Check sheet for the modelled part. Datum: model origin and axes. Units: mm. A direction names the side the tool comes from. Round coordinates to 2 decimals unless told otherwise and drop trailing zeros. Write each loop counter-clockwise with the first axis right and the second up, starting at its lowest first coordinate (ties: lowest second). Pieces come first, ordered by that corner, then holes. Notation, with made-up numbers: M 63.5,31.5 L 109.5,31.5 A21 ccw 109.5,52.5 Z; hole C 65.25,-23 d1. An arc over 180 degrees is marked long. One line per item, written item: value.
from build123d import *

# Parameters (mm, degrees)
F2_DEPTH = 3.175
F3_DEPTH = 3.175
F4_R     = 7.203715
F5_DEPTH = 25.4


with BuildPart() as f2:
    # F1 (on Front) → F2 (new body)
    with BuildSketch(Plane.XZ):
        with BuildLine():
            Line((-5.268215, -88.649482), (-5.268215, -81.455395))
            ThreePointArc((-5.268215, -81.455395), (0.311401, -67.985011), (13.781785, -62.405395))
            Line((13.781785, -62.405395), (20.131785, -62.405395))
            Line((20.131785, -62.405395), (20.131785, 79.52777))
            Line((20.131785, 79.52777), (7.431785, 79.52777))
            Line((7.431785, 79.52777), (7.431785, 70.944605))
            ThreePointArc((7.431785, 70.944605), (-5.63649, 39.464613), (-37.157186, 26.494822))
            Line((-37.157186, 26.494822), (-43.368766, 26.494822))
            Line((-43.368766, 26.494822), (-43.368215, 20.144822))
            add(Edge.make_bspline(
                [(-43.368215, 20.144822), (-17.968215, -15.569895), (-17.968215, -23.519904), (-17.968215, -81.455395)],
                knots=[0, 0, 0, 0, 104.727094, 104.727094, 104.727094, 104.727094], degree=3))
            Line((-17.968215, -81.455395), (-17.968215, -88.649482))
            Line((-17.968215, -88.649482), (-11.618215, -88.649482))
            Line((-11.618215, -88.649482), (-5.268215, -88.649482))
        make_face()
    extrude(amount=F2_DEPTH)

    # F0 (on Front) → F3 (cut)
    with BuildSketch(Plane.XZ):
        with BuildLine():
            Line((10.60685, -56.254837), (10.60685, 20.144395))
            Line((10.60685, 20.144395), (10.60685, 53.26673))
            ThreePointArc((10.60685, 53.26673), (9.14903, 49.749299), (7.43185, 46.350937))
            Line((7.43185, 46.350937), (7.43185, 20.144409))
            Line((7.43185, 20.144409), (7.43185, -56.862174))
            ThreePointArc((7.43185, -56.862174), (9.009679, -56.507945), (10.60685, -56.254837))
        make_face()
        with BuildLine():
            Line((4.25685, -57.909188), (4.25685, 20.144423))
            Line((4.25685, 20.144423), (4.25685, 41.329953))
            ThreePointArc((4.25685, 41.329953), (2.719376, 39.296806), (1.08185, 37.34334))
            Line((1.08185, 37.34334), (1.08185, 20.144436))
            Line((1.08185, 20.144436), (1.08185, -59.458573))
            ThreePointArc((1.08185, -59.458573), (2.64238, -58.628612), (4.25685, -57.909188))
        make_face()
        with BuildLine():
            Line((-2.09315, -61.62775), (-2.09315, 20.14445))
            Line((-2.09315, 20.14445), (-2.09315, 34.054215))
            ThreePointArc((-2.09315, 34.054215), (-3.651984, 32.638521), (-5.26815, 31.288645))
            Line((-5.26815, 31.288645), (-5.26815, 20.144463))
            Line((-5.26815, 20.144463), (-5.26815, -64.655097))
            ThreePointArc((-5.26815, -64.655097), (-3.74613, -63.072749), (-2.09315, -61.62775))
        make_face()
        with BuildLine():
            Line((-8.44315, -69.158896), (-8.44315, 20.144477))
            Line((-8.44315, 20.144477), (-8.44315, 28.94308))
            ThreePointArc((-8.44315, 28.94308), (-10.012262, 27.91739), (-11.61815, 26.950291))
            Line((-11.61815, 26.950291), (-11.61815, 20.14449))
            Line((-11.61815, 20.14449), (-11.618149, -81.455618))
            ThreePointArc((-11.618149, -81.455618), (-10.811594, -75.105618), (-8.44315, -69.158896))
        make_face()
        with BuildLine():
            Line((-14.79315, -22.322719), (-14.79315, 20.144504))
            Line((-14.79315, 20.144504), (-14.79315, 25.264087))
            ThreePointArc((-14.79315, 25.264087), (-16.368567, 24.530647), (-17.96815, 23.851521))
            Line((-17.96815, 23.851521), (-17.96815, 20.144518))
            Line((-17.96815, 20.144518), (-17.968287, -12.036756))
            Line((-17.968287, -12.036756), (-14.79315, -22.322719))
        make_face()
        with BuildLine():
            Line((-21.14315, -4.943635), (-21.14315, 20.144531))
            Line((-21.14315, 20.144531), (-21.14315, 22.68856))
            ThreePointArc((-21.14315, 22.68856), (-22.723067, 22.19717), (-24.31815, 21.757493))
            Line((-24.31815, 21.757493), (-24.31815, 20.144545))
            Line((-24.31815, 20.144545), (-24.31815, 0.903125))
            Line((-24.31815, 0.903125), (-21.14315, -4.943635))
        make_face()
        with BuildLine():
            Line((-27.49315, 6.121868), (-27.49315, 20.144558))
            Line((-27.49315, 20.144558), (-27.49315, 21.04534))
            ThreePointArc((-27.49315, 21.04534), (-29.076674, 20.76896), (-30.66815, 20.542819))
            Line((-30.66815, 20.542819), (-30.66815, 20.144572))
            Line((-30.66815, 20.144572), (-30.66815, 10.984366))
            Line((-30.66815, 10.984366), (-27.49315, 6.121868))
        make_face()
        with BuildLine():
            Line((-33.84315, 15.63159), (-33.84315, 20.144585))
            add(Edge.make_bspline(
                [(-33.84315, 20.243698), (-33.84315, 20.21066), (-33.84315, 20.177623), (-33.84315, 20.144585)],
                knots=[0, 0, 0, 0, 0.099112, 0.099112, 0.099112, 0.099112], degree=3))
            ThreePointArc((-33.84315, 20.243698), (-35.429797, 20.169219), (-37.017997, 20.144382))
            add(Edge.make_bspline(
                [(-37.017997, 20.144382), (-35.959714, 18.640118), (-34.901432, 17.135854), (-33.84315, 15.63159)],
                knots=[0.000266, 0.000266, 0.000266, 0.000266, 5.51796, 5.51796, 5.51796, 5.51796], degree=3))
        make_face()
    extrude(amount=F3_DEPTH, mode=Mode.SUBTRACT)

    # F4 (on Front) → F5 (cut)
    with BuildSketch(Plane.XZ):
        with Locations((-26.025116, 29.219549)):
            Circle(F4_R)
    extrude(amount=F5_DEPTH, mode=Mode.SUBTRACT)


solid = f2.part
Q1. Sectioned sample at D-D on z = 55. Enter the section's corners in (x, y) (3 decimals).
Completed:
outline: M 4.474,-3.175 L 20.132,-3.175 L 20.132,0 L 4.474,0 Z
Q2. Draft check along X on faces 1 (the flat face through (-7, 0, -4)), 2 (the flat face through (-2.093, -2, -14)), 3 (the flat face through (7.432, -2, 75)). Enter one of: pulls with the +X half, pulls with the -X half, needs draft (parallel to the pull), parting line crosses it, or undercut.
Completed:
face 1: needs draft
face 2: undercut
face 3: pulls with the -X half
Q3. Sectioned sample at A-A on x = 9. Enter the section's corners in (y, z) (3 decimals).
Completed:
outline: M -3.175,-63.015 L 0,-63.015 L 0,-56.51 L -3.175,-56.51 Z; M -3.175,49.428 L 0,49.428 L 0,79.528 L -3.175,79.528 Z
Q4. Depth check by flat-ended pin: P1, Ø1.6, axis at y = -1.5, z = -85.5, coming from the -X side; P2, Ø1, axis at y = -2.5, z = -5, coming from the -X side; P3, Ø1, axis at y = -1.5, z = -86.5, coming from the +X side. Enter the tip coordinate at first touch or a pass-through.
Completed:
P1: x = -17.97
P2: x = -27.72
P3: x = -5.27
Q5. Sectioned sample at B-B on y = -2.3. State how many separate pieces and enclosed holes the cut face has, and give its area (3 significant figures).
Completed:
separate pieces: 1
enclosed holes: 8
area: 4,030 mm^2
Q6. Scan lines: line 1 (X direction, y = -0.6, z = 34.5); line 2 (X direction, y = -0.5, z = -47); line 3 (X direction, y = -0.75, z = -33). Record each from-to range of solid material in increasing order. Write a range as [from, to].
Completed:
line 1: [-11.57, 1.08], [4.26, 7.43], [10.61, 20.13]
line 2: [-18.33, -11.62], [-8.44, -5.27], [-2.09, 1.08], [4.26, 7.43], [10.61, 20.13]
line 3: [-19.34, -11.62], [-8.44, -5.27], [-2.09, 1.08], [4.26, 7.43], [10.61, 20.13]
Q7. Access from +Z, -Z, +X, -X, +Y, -Y to the whole of each face (thin tool, end or side, straight path). Record for faces 4 (the cylindrical face through (0.2, -1.6, -68.1)), 5 (the flat face through (4.257, -2, -9)).
Completed:
face 4: -Z, +X, +Y, -Y
face 5: +Y, -Y
